Design review of the part built by this model. Coordinates are the model's own, in mm. A direction names the side the tool comes from. Coordinates: 2 decimals unless noted, no trailing zeros. Order: outer loops, then holes, each group sorted by start corner. A loop starts at its lowest first (then second) coordinate and runs counter-clockwise, first axis right, second up. Notation, with made-up numbers: M -9,39.25 L 40,39.25 A25 cw 40,77.25 Z; hole C 25,8.25 d8. An arc over 180 degrees is marked long. Use CSV: the item, a comma, the result in double quotes.
```python
from build123d import *

# Parameters (mm, degrees)
F1_DEPTH  = 130
F3_DEPTH  = 125
F6_DEPTH  = 10
F7_DEPTH  = 10
F9_DEPTH  = 5
F10_R     = 10
F11_DEPTH = 5.001
F12_R     = 10
F13_DEPTH = 5.001
F14_R     = 4
F15_DEPTH = 130.001
F16_ANGLE = 180


with BuildPart() as f1:
    # F0 (on Top) → F1 (new body)
    with BuildSketch(Plane.XY):
        Polygon((0, 60), (0, 0), (60, 0), (60, 15), (15, 60), align=None)
    extrude(amount=F1_DEPTH)

    # F2 (on face) → F3 (cut)
    with BuildSketch(Plane.XY.offset(130)):
        Polygon((15, 15), (60, 15), (15, 60), align=None)
    extrude(amount=-F3_DEPTH, mode=Mode.SUBTRACT)

    # F5 (on face) → F6 (cut)
    with BuildSketch(Plane.YZ.offset(15)):
        with BuildLine():
            Line((52.5, 25), (52.5, 105))
            ThreePointArc((52.5, 105), (37.5, 120), (22.5, 105))
            Line((22.5, 105), (22.5, 25))
            ThreePointArc((22.5, 25), (37.5, 10), (52.5, 25))
        make_face()
    extrude(amount=-F6_DEPTH, mode=Mode.SUBTRACT)

    # F4 (on face) → F7 (cut)
    with BuildSketch(Plane(origin=(0, 15, 0), x_dir=(-1, 0, 0), z_dir=(0, 1, 0))):
        with BuildLine():
            Line((-22.5, 25), (-22.5, 105))
            ThreePointArc((-22.5, 105), (-37.5, 120), (-52.5, 105))
            Line((-52.5, 105), (-52.5, 25))
            ThreePointArc((-52.5, 25), (-37.5, 10), (-22.5, 25))
        make_face()
    extrude(amount=-F7_DEPTH, mode=Mode.SUBTRACT)

    # F8 (on face) → F9 (join)
    with BuildSketch(Plane.XY.offset(130)):
        Polygon((15, 15), (60, 15), (15, 60), align=None)
    extrude(amount=-F9_DEPTH)

    # F10 (on face) → F11 (cut, through all)
    with BuildSketch(Plane(origin=(0, 5, 0), x_dir=(-1, 0, 0), z_dir=(0, 1, 0))):
        with Locations((-37.5, 105)):
            Circle(F10_R)
        with Locations((-37.5, 65)):
            Circle(F10_R)
        with Locations((-37.5, 25)):
            Circle(F10_R)
    extrude(amount=-F11_DEPTH, mode=Mode.SUBTRACT)

    # F12 (on face) → F13 (cut, through all)
    with BuildSketch(Plane.YZ.offset(5)):
        with Locations((37.5, 105)):
            Circle(F12_R)
        with Locations((37.5, 65)):
            Circle(F12_R)
        with Locations((37.5, 25)):
            Circle(F12_R)
    extrude(amount=-F13_DEPTH, mode=Mode.SUBTRACT)

    # F14 (on face) → F15 (cut, through all)
    with BuildSketch(Plane.XY.offset(130)):
        with Locations((40.686292, 23)):
            Circle(F14_R)
        with Locations((23, 40.686292)):
            Circle(F14_R)
    extrude(amount=-F15_DEPTH, mode=Mode.SUBTRACT)


with BuildPart() as f1_1:
    # F16: moved
    add(f1.part.rotate(Axis((0, 0, 65), (0, 0, 1)), F16_ANGLE))


solid = f1_1.part
```
(1) Add section B-B on y = -55. State the section outline as (x, z) points.
The answers:
outline,"M -20,0 L 0,0 L 0,130 L -20,130 L -20,125 L -15,125 L -15,5 L -20,5 Z"
(2) Add section C-C on z = 46.5. State the section outline as (x, y) points, and give its area (3 significant figures).
The answers:
outline,"M -60,-15 L -52.5,-15 L -52.5,-5 L -22.5,-5 L -22.5,-15 L -15,-15 L -15,-22.5 L -5,-22.5 L -5,-52.5 L -15,-52.5 L -15,-60 L 0,-60 L 0,0 L -60,0 Z"
area,"975 mm2"
(3) Add section A-A on z = 65. State the section outline as (x, y) points, and give its area (3 significant figures).
The answers:
outline,"M -60,-15 L -52.5,-15 L -52.5,-5 L -47.5,-5 L -47.5,0 L -60,0 Z; M -27.5,-5 L -22.5,-5 L -22.5,-15 L -15,-15 L -15,-22.5 L -5,-22.5 L -5,-27.5 L 0,-27.5 L 0,0 L -27.5,0 Z; M -15,-60 L 0,-60 L 0,-47.5 L -5,-47.5 L -5,-52.5 L -15,-52.5 Z"
area,"775 mm2"
(4) The part is to be moulded in two halves that separate along Y. For faces 1 (the face through (-47.49, -2.53, 65.44)), 2 (the face through (-23, 0, 64)), 3 (the face through (-10.07, -37.17, 10.004)), 4 (the face through (-22, -15, 66)), say which applies: pulls with the +Y half, pulls with the -Y half, needs draft (parallel to the pull), parting line crosses it, or undercut.
The answers:
face 1,"needs draft"
face 2,"pulls with the +Y half"
face 3,"undercut"
face 4,"pulls with the -Y half"
(5) Wall thickness on probe 1 along Z at (x, y) = (-3, -37); probe 2 along Z at (x, y) = (-22.5, -22); probe 3 along Y at (x, z) = (-50, 88): over which ranges is each line inside the solid? List them lowest first.
The answers:
probe 1,"z = 0 to 15.01, 34.99 to 55.01, 74.99 to 95.01, 114.99 to 130"
probe 2,"z = 0 to 5, 125 to 130"
probe 3,"y = -5 to 0"
(6) Clearance check with flat-ended pins moving along their axes: P1, Ø2, axis at y = -33, z = 114.5, coming from the -X side; P2, Ø16, axis at x = -37.5, z = 65, coming from the +Y side; P3, Ø4, axis at x = -23, z = 101, coming from the -Y side; P4, Ø3, axis at x = -26.5, z = 30.5, coming from the -Y side. State where each tip first meets the part, or that it passes through.
The answers:
P1,"stops at x = -5"
P2,"passes through"
P3,"stops at y = -15"
P4,"stops at y = -5"
(7) Add section D-D on y = -21. State the section outline as (x, z) points, and give its area (3 significant figures).
The answers:
outline,"M -54,0 L -44.15,0 L -44.15,5 L -54,5 Z; M -54,125 L -44.15,125 L -44.15,130 L -54,130 Z; M -37.22,0 L 0,0 L 0,130 L -37.22,130 L -37.22,125 L -15,125 L -15,5 L -37.22,5 Z"
area,"2,270 mm2"
(8) For faces 5 (the face through (-27, -28, 125)), 6 (the face through (-10, -22.5, 66)), 7 (the face through (-2.535, -36.198, 34.915)), 8 (the face through (-38.802, -2.535, 114.915)), 9 (the face through (-52.5, -10, 66)), list the 3-axis set-ups (+Z, -Z, +X, -X, +Y, -Y) from which the entire face can be reached by the end or side of a thin tool; tool diameter is ignored.
The answers:
face 5,"-X, -Y"
face 6,"-X"
face 7,"+X, -X"
face 8,"+Y, -Y"
face 9,"-Y"
